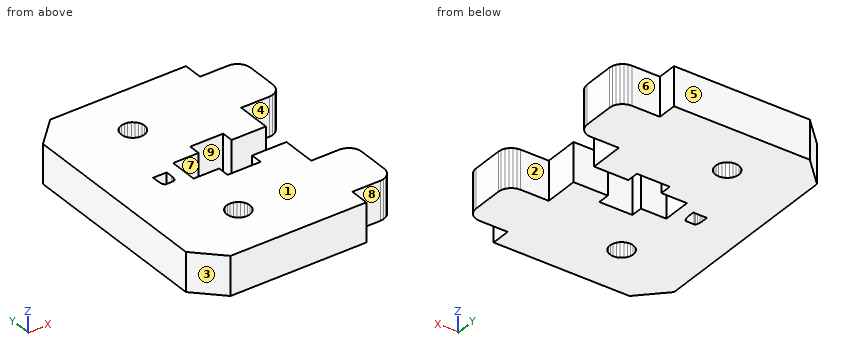
from build123d import *

# Parameters (mm, degrees)
BOSS_EXTRUDE1_DEPTH = 6


with BuildPart() as part:
    # Sketch1 → Boss-Extrude1 (new body)
    with BuildSketch(Plane.XY):
        Polygon((316.255247905, 240.964803396), (315.841034343, 241.282640641), (315.358672433, 241.482441486), (314.841034343, 241.550589833), (310.491036452, 241.550589833), (310.491036452, 246.850587088), (305.19103763, 246.850587088), (305.19103763, 245.050588856), (300.091039865, 245.050588856), (300.091039865, 246.850587088), (296.141040043, 246.850587088), (296.141040043, 251.25059176), (300.091039865, 251.25059176), (300.091039865, 253.050589992), (305.19103763, 253.050589992), (305.19103763, 251.25059176), (310.491036452, 251.25059176), (310.491036452, 256.550583767), (314.841034343, 256.550583767), (315.358672433, 256.618732114), (315.841034343, 256.818532959), (316.255247905, 257.136370204), (316.57308515, 257.550583767), (316.772885995, 258.032945676), (316.841034343, 258.550583767), (316.841034343, 263.350579732), (316.772885995, 263.868217822), (316.57308515, 264.350579732), (316.255247905, 264.764793294), (315.841034343, 265.082630539), (315.358672433, 265.282431384), (314.841034343, 265.350579732), (310.491036452, 265.350579732), (310.491036452, 268.350579732), (289.491036452, 268.350579732), (285.491036452, 264.350579732), (285.491036452, 233.750595391), (289.491036452, 229.750595391), (310.491036452, 229.750595391), (310.491036452, 232.750595391), (314.841034343, 232.750595391), (315.358672433, 232.818743738), (315.841034343, 233.018544583), (316.255247905, 233.336381829), (316.57308515, 233.750595391), (316.772885995, 234.232957301), (316.841034343, 234.750595391), (316.841034343, 239.550589833), (316.772885995, 240.068227923), (316.57308515, 240.550589833), align=None)
        Polygon((296.491036452, 235.950595391), (296.02516217, 236.011928904), (295.591036452, 236.191749664), (295.218244245, 236.477803185), (294.932190725, 236.850595391), (294.752369964, 237.28472111), (294.691036452, 237.750595391), (294.752369964, 238.216469672), (294.932190725, 238.650595391), (295.218244245, 239.023387597), (295.591036452, 239.309441118), (296.02516217, 239.489261878), (296.491036452, 239.550595391), (296.956910733, 239.489261878), (297.391036452, 239.309441118), (297.763828658, 239.023387597), (298.049882178, 238.650595391), (298.229702939, 238.216469672), (298.291036452, 237.750595391), (298.229702939, 237.28472111), (298.049882178, 236.850595391), (297.763828658, 236.477803185), (297.391036452, 236.191749664), (296.956910733, 236.011928904), align=None, mode=Mode.SUBTRACT)
        Polygon((292.167294345, 248.521745899), (292.136860132, 248.95490496), (292.136860132, 249.972673633), (292.137050681, 249.972673633), (294.228561733, 249.972673633), (294.228561733, 248.95490496), (294.193435256, 248.521745899), (294.088055826, 248.158815973), (293.932728797, 247.912954455), (293.84394944, 247.851489075), (293.747759523, 247.831000615), (292.580314782, 247.831000615), (292.58017187, 247.831000615), (292.485290658, 247.851455341), (292.485134177, 247.851489075), (292.399859132, 247.912954455), (292.258596985, 248.158815973), align=None, mode=Mode.SUBTRACT)
        Polygon((295.218244245, 259.077787526), (294.932190725, 259.450579732), (294.752369964, 259.884705451), (294.691036452, 260.350579732), (294.752369964, 260.816454013), (294.932190725, 261.250579732), (295.218244245, 261.623371938), (295.591036452, 261.909425459), (296.02516217, 262.089246219), (296.491036452, 262.150579732), (296.956910733, 262.089246219), (297.391036452, 261.909425459), (297.763828658, 261.623371938), (298.049882178, 261.250579732), (298.229702939, 260.816454013), (298.291036452, 260.350579732), (298.229702939, 259.884705451), (298.049882178, 259.450579732), (297.763828658, 259.077787526), (297.391036452, 258.791734005), (296.956910733, 258.611913244), (296.491036452, 258.550579732), (296.02516217, 258.611913244), (295.591036452, 258.791734005), align=None, mode=Mode.SUBTRACT)
    extrude(amount=BOSS_EXTRUDE1_DEPTH)


solid = part.part
Check sheet for the modelled part. Datum: model origin and axes. Units: mm. Face numbers are marked on the shaded views. A direction names the side the tool comes from. Give positions to 0.01 mm unless a question says otherwise; leave off trailing zeros. Loops run counter-clockwise (first coordinate to the right, second up) from the corner with the lowest first, then second, coordinate; pieces in that order, holes last. Notation, with made-up numbers: M 67,69.5 L 87,69.5 A31 cw 87,98.5 Z; hole C -13,41 d8. An arc over 180 degrees is marked long. Use a Markdown table: item, result. Add a question column.
Q1. Mould release check, pull along Y, two halves, no side actions. Record for the marked faces 1, 2, 3 and 4: pulls with the +Y half, pulls with the -Y half, needs draft (parallel to the pull), parting line crosses it, or undercut.
Q2. Sectioned sample at A-A, the plane x = 312. Record the cut outline in (y, z).
Q3. Scan lines: line 1 along Y through (x, z) = (296.5, 5.2); line 2 along Y through (x, z) = (313, 2.3); line 3 along Y through (x, z) = (310, 2.05). Record each from-to range of solid material in increasing order. Write a range as [from, to].
Q4. Sectioned sample at B-B, the plane y = 245.5. Record the cut outline in (x, z), then the cut area to 3 significant figures.
Q5. Sectioned sample at D-D, the plane y = 250.5. Record the cut outline in (x, z), then the cut area to 3 significant figures.
Q6. Go/stop test with flat-tipped pins: pin 1 (0.5 mm diameter, centred on y = 246, z = 4, fed in from +X); pin 2 (1.3 mm diameter, centred on y = 248.5, z = 3, fed in from +X); pin 3 (2 mm diameter, centred on x = 312.5, z = 3.5, fed in from +Y). Record where each tip stops, or that it passes through.
Q7. Tool access check on the marked faces 5, 6, 7, 8 and 9. Record the directions out of +Z, -Z, +X, -X, +Y, -Y that give a thin tool (end or side, any length) a straight path to the whole face; none if there is none.
Q8. Sectioned sample at C-C, the plane z = 5.05. Give the number of separate pieces and of enclosed holes in the cut face, then the cut area to 3 significant figures.
Verdict:
| question | item | result |
|---|---|---|
| 1 | face 1 | needs draft |
| 1 | face 2 | undercut |
| 1 | face 3 | pulls with the -Y half |
| 1 | face 4 | undercut |
| 2 | outline | M 232.75,0 L 241.55,0 L 241.55,6 L 232.75,6 Z; M 256.55,0 L 265.35,0 L 265.35,6 L 256.55,6 Z |
| 3 | line 1 | [229.75, 235.95], [239.55, 246.85], [251.25, 258.55], [262.15, 268.35] |
| 3 | line 2 | [232.75, 241.55], [256.55, 265.35] |
| 3 | line 3 | [229.75, 246.85], [251.25, 268.35] |
| 4 | outline | M 285.49,0 L 300.09,0 L 300.09,6 L 285.49,6 Z; M 305.19,0 L 310.49,0 L 310.49,6 L 305.19,6 Z |
| 4 | area | 119 mm^2 |
| 5 | outline | M 285.49,0 L 296.14,0 L 296.14,6 L 285.49,6 Z |
| 5 | area | 63.9 mm^2 |
| 6 | pin 1 | x = 310.49 |
| 6 | pin 2 | x = 296.14 |
| 6 | pin 3 | y = 265.35 |
| 7 | face 5 | +Z, -Z, +X, -X, +Y |
| 7 | face 6 | +Z, -Z, +X, +Y |
| 7 | face 7 | +Z, -Z, +X |
| 7 | face 8 | +Z, -Z, +X, -Y |
| 7 | face 9 | +Z, -Z |
| 8 | separate pieces | 1 |
| 8 | enclosed holes | 3 |
| 8 | area | 951 mm^2 |
